The drawing under review shows one solid part. Ordinate dimensions are in mm from its lowest x, y, z. A direction names the side the tool comes from. Round coordinates to 2 decimals unless told otherwise and drop trailing zeros. Loops run counter-clockwise (first coordinate to the right, second up) from the corner with the lowest first, then second, coordinate; pieces in that order, holes last. Notation, with made-up numbers: M 12.5,-28 L 62.5,-28 A19 ccw 62.5,-11 Z; hole C 80.25,-24.75 d1. An arc over 180 degrees is marked long. Use a Markdown table: item, result.
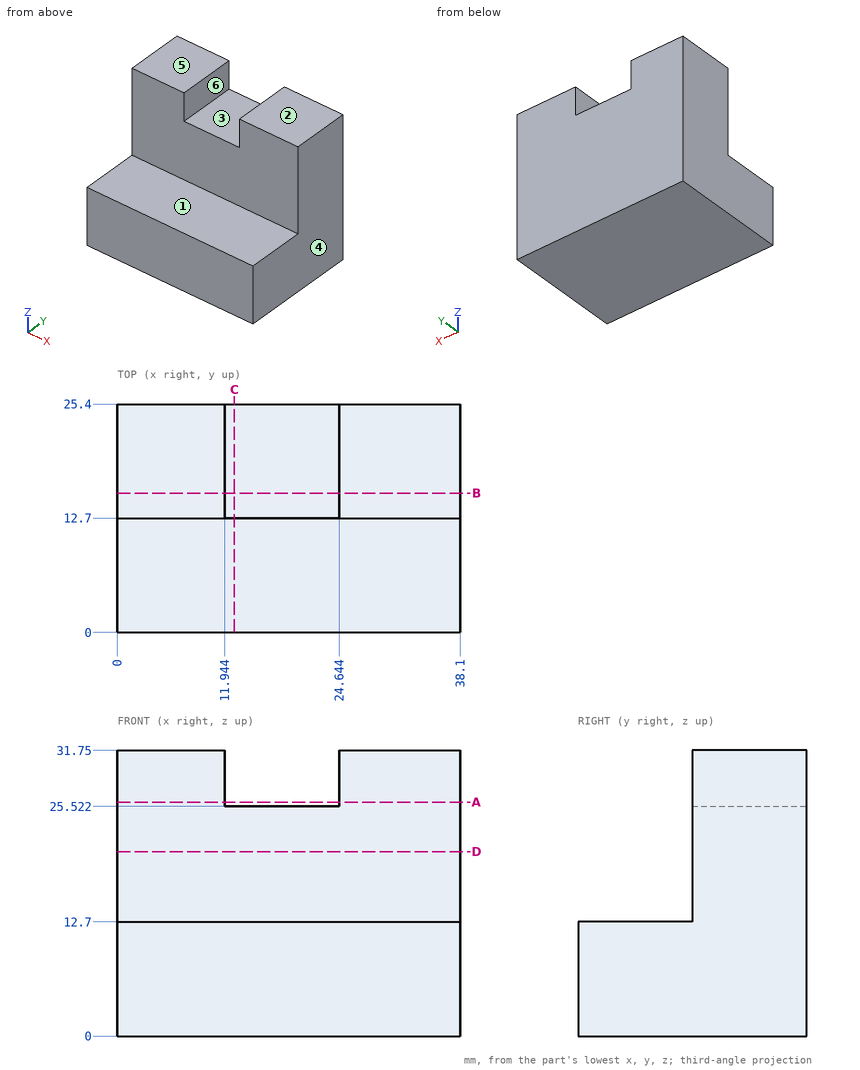
1. Machinability: for the marked faces 1, 2 and 3, which of the approach directions +Z, -Z, +X, -X, +Y, -Y give a long, thin tool a straight path to every point of the face, cutting with its end or side? Answer none if there is none.
Check values:
| item | result |
|---|---|
| face 1 | +Z, +X, -X, -Y |
| face 2 | +Z, +X, -X, +Y, -Y |
| face 3 | +Z, +Y, -Y |
2. Insertion check: pin 1 (4 mm diameter, centred on x = 18.5, y = 17, fed in from +Z); pin 2 (1.5 mm diameter, centred on x = 10, z = 27.5, fed in from -Y). Each pin has a flat end and moves straight along its axis. Give the tip position at first contact, or say it passes through.
Check values:
| item | result |
|---|---|
| pin 1 | stops at z = 25.52 |
| pin 2 | stops at y = 12.7 |
3. The part is to be moulded in two halves that separate along X. For the marked faces 4, 5 and 6, say which applies: pulls with the +X half, pulls with the -X half, needs draft (parallel to the pull), parting line crosses it, or undercut.
Check values:
| item | result |
|---|---|
| face 4 | pulls with the +X half |
| face 5 | needs draft |
| face 6 | undercut |
4. Take a section at A-A on z = 26. Give the boundary of the cut face in (x, y).
Check values:
| item | result |
|---|---|
| outline | M 0,12.7 L 11.94,12.7 L 11.94,25.4 L 0,25.4 Z; M 24.64,12.7 L 38.1,12.7 L 38.1,25.4 L 24.64,25.4 Z |
5. Take a section at C-C on x = 13. Give the boundary of the cut face in (y, z), and give its area (3 significant figures).
Check values:
| item | result |
|---|---|
| outline | M 0,0 L 25.4,0 L 25.4,25.52 L 12.7,25.52 L 12.7,12.7 L 0,12.7 Z |
| area | 485 mm² |
6. Wall thickness on line 1 along Y through (x, z) = (21, 22); line 2 along Z through (x, y) = (20, 23); line 3 along Z through (x, y) = (4.5, 6): over which ranges is each line inside the solid? List them lowest first. Write a range as from..to.
Check values:
| item | result |
|---|---|
| line 1 | y = 12.7..25.4 |
| line 2 | z = 0..25.52 |
| line 3 | z = 0..12.7 |
7. Take a section at B-B on y = 15.5. Give the boundary of the cut face in (x, z).
Check values:
| item | result |
|---|---|
| outline | M 0,0 L 38.1,0 L 38.1,31.75 L 24.64,31.75 L 24.64,25.52 L 11.94,25.52 L 11.94,31.75 L 0,31.75 Z |
8. Take a section at D-D on z = 20.5. Give the boundary of the cut face in (x, y), and give its area (3 significant figures).
Check values:
| item | result |
|---|---|
| outline | M 0,12.7 L 38.1,12.7 L 38.1,25.4 L 0,25.4 Z |
| area | 484 mm² |
